```python
from build123d import *

# Parameters (mm, degrees)
SKETCH1_R           = 5
SKETCH1_R_2         = 3
BOSS_EXTRUDE1_DEPTH = 2
SKETCH2_R           = 5
BOSS_EXTRUDE2_DEPTH = 2
SKETCH3_R           = 0.5
CUT_EXTRUDE1_DEPTH  = 5
BOSS_EXTRUDE3_DEPTH = 4


with BuildPart() as part:
    # Sketch1 → Boss-Extrude1 (new body)
    with BuildSketch(Plane(origin=(0, 0, 0), x_dir=(1, 0, 0), z_dir=(0, 1, 0))):
        with Locations((-1, 0)):
            Circle(SKETCH1_R)
        Circle(SKETCH1_R_2, mode=Mode.SUBTRACT)
    extrude(amount=BOSS_EXTRUDE1_DEPTH)

    # Sketch2 → Boss-Extrude2 (add)
    with BuildSketch(Plane(origin=(0, 2, 0), x_dir=(1, 0, 0), z_dir=(0, 1, 0))):
        with Locations((-1, 0)):
            Circle(SKETCH2_R)
    extrude(amount=BOSS_EXTRUDE2_DEPTH)

    # Sketch3 → Cut-Extrude1 (cut, through all)
    with BuildSketch(Plane.XZ):
        with Locations((0, 3.75)):
            Circle(SKETCH3_R)
        with Locations((0, -3.75)):
            Circle(SKETCH3_R)
    extrude(amount=-CUT_EXTRUDE1_DEPTH, mode=Mode.SUBTRACT)

    # Sketch4 → Boss-Extrude3 (add)
    with BuildSketch(Plane.XZ):
        with BuildLine():
            ThreePointArc((-2, 2.236067977), (-3, 0), (-2, -2.236067977))
            Line((-2, -2.236067977), (-2, 2.236067977))
        make_face()
    extrude(amount=-BOSS_EXTRUDE3_DEPTH)


solid = part.part
```
Could you check a few things on this model? Use its own coordinates, in mm. A direction names the side the tool comes from. Round coordinates to 2 decimals unless told otherwise and drop trailing zeros. Write each loop counter-clockwise with the first axis right and the second up, starting at its lowest first coordinate (ties: lowest second). Pieces come first, ordered by that corner, then holes.
(1) Suppose I cut it at B-B on x = 2. Write out the boundary of the cut face in (y, z), and give its area (3 significant figures).
Findings below:
outline: (0, -4) - (4, -4) - (4, 4) - (0, 4) - (0, 2.24) - (2, 2.24) - (2, -2.24) - (0, -2.24) - close
area: 23.1 mm2
(2) Suppose I cut it at C-C on y = 0.55. Write out the boundary of the cut face in (x, z).
Findings below:
outline: circle Ø10 at (-1, 0); hole (-2, -2.24) arc R3 ccw (long way) to (-2, 2.24) - close; hole circle Ø1 at (0, -3.75); hole circle Ø1 at (0, 3.75)
(3) Suppose I cut it at A-A on z = 3.5. Write out the boundary of the cut face in (x, y).
Findings below:
outline: (-4.57, 0) - (-0.43, 0) - (-0.43, 4) - (-4.57, 4) - close; (0.43, 0) - (2.57, 0) - (2.57, 4) - (0.43, 4) - close
(4) If I drill on probe 1 along Z at (x, y) = (0, 2.8); probe 2 along Z at (x, y) = (0, 1.7); probe 3 along X at (y, z) = (1.1, 0), over which ranges is the centre line in solid material (lowest first)?
Findings below:
probe 1: z = -4.9 to -4.25, -3.25 to 3.25, 4.25 to 4.9
probe 2: z = -4.9 to -4.25, -3.25 to -3, 3 to 3.25, 4.25 to 4.9
probe 3: x = -6 to -2, 3 to 4
(5) Thinking about a two-plate mould opening in X: for faces 1 (the face through (-2.08, 1.97, 4.88)), 2 (the face through (-2.2, 0, 0.1)), 3 (the face through (0, 2, 0)), which applies, +X half, -X half, draft (parallel to the pull), parting line (faces both ways), or undercut?
Findings below:
face 1: parting line
face 2: draft
face 3: undercut
(6) For pin 1 (2 mm diameter, centred on x = 1.5, y = 3, fed in from +Z); pin 2 (1.5 mm diameter, centred on x = 0.5, z = 0.5, fed in from -Y); pin 3 (4 mm diameter, centred on x = 0, z = -3.5, fed in from -Y); pin 4 (1 mm diameter, centred on y = 1.5, z = -3.5, fed in from -X), each with a flat end and sliding along its axis, tell me the tip position at first contact or that it passes through.
Findings below:
pin 1: stops at z = 4.77
pin 2: stops at y = 2
pin 3: stops at y = 0
pin 4: stops at x = -5
(7) Which directions (+Z, -Z, +X, -X, +Y, -Y) give clear straight access to the entire face, cutting with the end or side of a thin tool? Please do faces 4 (the face through (3, 1, 0)), 5 (the face through (-0.065, 1.972, 4.246)).
Findings below:
face 4: -Y
face 5: +Y, -Y
(8) Suppose I cut it at D-D on z = 0. Write out the boundary of the cut face in (x, y), and give its area (3 significant figures).
Findings below:
outline: (-6, 0) - (-2, 0) - (-2, 2) - (3, 2) - (3, 0) - (4, 0) - (4, 4) - (-6, 4) - close
area: 30.0 mm2
